Part model, mm, in its own coordinate system. A direction names the side the tool comes from. Coordinates: 2 decimals unless noted, no trailing zeros. Order: outer loops, then holes, each group sorted by start corner. A loop starts at its lowest first (then second) coordinate and runs counter-clockwise, first axis right, second up.
```python
from build123d import *

# Parameters (mm, degrees)
SKETCH1_W                = 27.2
SKETCH1_H                = 10
BOSS_EXTRUDE1_DEPTH      = 34.6
CUT_EXTRUDE1_DEPTH       = 1
CUT_EXTRUDE1_DEPTH_BACK  = 34.6
CHAMFER1_SIZE            = 0.7
M3_CLEARANCE_HOLE1_D     = 3.4
M3_CLEARANCE_HOLE1_DEPTH = 5
M3_CLEARANCE_HOLE1_TIP   = 1.021463052
SKETCH7_W                = 27.2
SKETCH7_H                = 5
CUT_EXTRUDE2_DEPTH       = 0.5
SKETCH8_W                = 5
SKETCH8_H                = 9.5
CUT_EXTRUDE3_DEPTH       = 0.5


with BuildPart() as part:
    # Sketch1 → Boss-Extrude1 (new body)
    with BuildSketch(Plane.XY):
        Rectangle(SKETCH1_W, SKETCH1_H)
    extrude(amount=BOSS_EXTRUDE1_DEPTH)

    # Sketch2 → Cut-Extrude1 (cut, two sides)
    with BuildSketch(Plane.XY.offset(34.6)) as cut_extrude1_sk:
        Polygon((-5.55, -3), (-6.05, -3.5), (-6.05, -5), (6.05, -5), (6.05, -3.5), (5.55, -3), (3.95, -3), (3.95, -1.4), (5.55, -1.4), (6.05, -0.9), (6.05, 0), (5.55, 0.5), (-5.55, 0.5), (-6.05, 0), (-6.05, -0.9), (-5.55, -1.4), (-3.95, -1.4), (-3.95, -3), align=None)
    extrude(amount=CUT_EXTRUDE1_DEPTH, mode=Mode.SUBTRACT)
    extrude(cut_extrude1_sk.sketch, amount=-CUT_EXTRUDE1_DEPTH_BACK, mode=Mode.SUBTRACT)

    # Chamfer1
    chamfer1_edges = [part.edges().sort_by_distance(p)[0] for p in [
        (-3.95, -3, 17.3),
        (3.95, -3, 17.3),
        (3.95, -1.4, 17.3),
        (-3.95, -1.4, 17.3),
    ]]
    chamfer(chamfer1_edges, length=CHAMFER1_SIZE)

    # M3 Clearance Hole1
    with Locations(Plane(origin=(0, 5, 0), x_dir=(1, 0, 0), z_dir=(0, 1, 0))):
        with Locations((-10, -24.8), (-10, -9.8), (10, -9.8), (10, -24.8)):
            Hole(M3_CLEARANCE_HOLE1_D / 2, depth=M3_CLEARANCE_HOLE1_DEPTH)
            with Locations((0, 0, -(M3_CLEARANCE_HOLE1_DEPTH + M3_CLEARANCE_HOLE1_TIP / 2))):  # 118° drill point
                Cone(0, M3_CLEARANCE_HOLE1_D / 2, M3_CLEARANCE_HOLE1_TIP, mode=Mode.SUBTRACT)

    # Sketch7 → Cut-Extrude2 (cut)
    with BuildSketch(Plane(origin=(0, 5, 0), x_dir=(1, 0, 0), z_dir=(0, 1, 0))):
        with Locations((0, -32.1)):
            Rectangle(SKETCH7_W, SKETCH7_H)
        with Locations((0, -2.5)):
            Rectangle(SKETCH7_W, SKETCH7_H)
    extrude(amount=-CUT_EXTRUDE2_DEPTH, mode=Mode.SUBTRACT)

    # Sketch8 → Cut-Extrude3 (cut)
    with BuildSketch(Plane(origin=(13.6, 0, 0), x_dir=(0, 0, -1), z_dir=(1, 0, 0))):
        with Locations((-32.1, -0.25)):
            Rectangle(SKETCH8_W, SKETCH8_H)
        with Locations((-2.5, -0.25)):
            Rectangle(SKETCH8_W, SKETCH8_H)
    cut_extrude3 = extrude(amount=-CUT_EXTRUDE3_DEPTH, mode=Mode.SUBTRACT)

    # Mirror1: Cut-Extrude3 across plane
    add(cut_extrude3.mirror(Plane(origin=(0, 0, 0), x_dir=(0, 0, 1), z_dir=(1, 0, 0))), mode=Mode.SUBTRACT)


solid = part.part
```
(1) Tool access for faces 1 (the face through (9.086, 2.465, 8.367)), 2 (the face through (-13.1, 0, 32)), 3 (the face through (-5, -3, 18)), 4 (the face through (0, 4.5, 32)): list every direction of +Z, -Z, +X, -X, +Y, -Y with a clear straight run to the whole face (end or side of a thin tool).
(2) Slice it at A-A, the plane y = -4. Give the cut face in (x, z).
(3) Probe line 1 (Z direction, x = 10, y = 1.8); line 2 (X direction, y = 2.5, z = 24.8); line 3 (X direction, y = -0.5, z = 29). List the from-to ranges inside material, lowest first.
(4) Slice it at B-B, the plane y = 3.5. Give the cut face in (x, z).
(5) Drop flat-ended pins along their axis: pin 1 (1 mm diameter, centred on x = -5.5, z = 14, fed in from -Y); pin 2 (1.5 mm diameter, centred on x = -1.5, z = 31.5, fed in from +Y); pin 3 (2 mm diameter, centred on x = -10, z = 24.8, fed in from +Y). Give the stop position or say it passes through.
(6) Slice it at D-D, the plane z = 15.5. Give the cut face in (x, y), then the cut area to 3 significant figures.
(7) Pull direction Z, two halves, no side cores. Call faces 5 (the face through (0, 1, 0)), 6 (the face through (-6.05, -4, 18)), 7 (the face through (0, 1, 34.6)), 8 (the face through (-10.038, -0.844, 9.507)): +Z half, -Z half, draft (parallel to the pull), parting line (faces both ways), or undercut.
(8) Slice it at C-C, the plane x = -2. Give the cut face in (y, z).
Here are the results:
1. face 1: +Y
1. face 2: +Z, -X, +Y, -Y
1. face 3: +Z, -Z, -Y
1. face 4: +Z, +X, -X, +Y
2. outline: (-13.6, 5) - (-13.1, 5) - (-13.1, 0) - (-6.05, 0) - (-6.05, 34.6) - (-13.1, 34.6) - (-13.1, 29.6) - (-13.6, 29.6) - close; (6.05, 0) - (13.1, 0) - (13.1, 5) - (13.6, 5) - (13.6, 29.6) - (13.1, 29.6) - (13.1, 34.6) - (6.05, 34.6) - close
3. line 1: z = 0 to 8.1, 11.5 to 23.1, 26.5 to 34.6
3. line 2: x = -13.6 to -11.7, -8.3 to 8.3, 11.7 to 13.6
3. line 3: x = -13.6 to -6.05, 6.05 to 13.6
4. outline: (-13.6, 5) - (-13.1, 5) - (-13.1, 0) - (13.1, 0) - (13.1, 5) - (13.6, 5) - (13.6, 29.6) - (13.1, 29.6) - (13.1, 34.6) - (-13.1, 34.6) - (-13.1, 29.6) - (-13.6, 29.6) - close; hole circle Ø3.4 at (-10, 9.8); hole circle Ø3.4 at (-10, 24.8); hole circle Ø3.4 at (10, 9.8); hole circle Ø3.4 at (10, 24.8)
5. pin 1: stops at y = -3.45
5. pin 2: stops at y = 4.5
5. pin 3: stops at y = -0.42
6. outline: (-13.6, -5) - (-6.05, -5) - (-6.05, -3.5) - (-5.55, -3) - (-4.65, -3) - (-3.95, -2.3) - (-3.95, -2.1) - (-4.65, -1.4) - (-5.55, -1.4) - (-6.05, -0.9) - (-6.05, 0) - (-5.55, 0.5) - (5.55, 0.5) - (6.05, 0) - (6.05, -0.9) - (5.55, -1.4) - (4.65, -1.4) - (3.95, -2.1) - (3.95, -2.3) - (4.65, -3) - (5.55, -3) - (6.05, -3.5) - (6.05, -5) - (13.6, -5) - (13.6, 5) - (-13.6, 5) - close
6. area: 212 mm2
7. face 5: -Z half
7. face 6: draft
7. face 7: +Z half
7. face 8: undercut
8. outline: (0.5, 0) - (4.5, 0) - (4.5, 5) - (5, 5) - (5, 29.6) - (4.5, 29.6) - (4.5, 34.6) - (0.5, 34.6) - close
